from build123d import *

# Parameters (mm, degrees)
BOX019_W               = 120
BOX019_H               = 30
BOX019_DEPTH           = 120
CYLINDER075_R          = 2.5
CYLINDER075_DEPTH      = 10
CYLINDER076_R          = 2.5
CYLINDER076_DEPTH      = 10
CYLINDER077_R          = 2.5
CYLINDER077_DEPTH      = 10
CYLINDER078_R          = 2.5
CYLINDER078_DEPTH      = 10
CYLINDER074_R          = 2.5
CYLINDER074_DEPTH      = 10
CYLINDER079_R          = 2.5
CYLINDER079_DEPTH      = 10
BOX016_W               = 240
BOX016_H               = 5
BOX016_DEPTH           = 24
BOX017_W               = 140
BOX017_H               = 5
BOX017_DEPTH           = 38
BOX018_W               = 140
BOX018_H               = 5
BOX018_DEPTH           = 77
CUT010_PLACEMENT_ANGLE = 270


with BuildPart() as gatewaycut002:
    # Box019 → Box019 (new body)
    with BuildSketch(Plane(origin=(-75, -3.2, -111), x_dir=(1, 0, 0), z_dir=(0, 0, 1))):
        with Locations((60, 15)):
            Rectangle(BOX019_W, BOX019_H)
    extrude(amount=BOX019_DEPTH)


with BuildPart() as cylinder075:
    # Cylinder075 → Cylinder075 (new body)
    with BuildSketch(Plane(origin=(115, 0, -31), x_dir=(1, 0, 0), z_dir=(0, -1, 0))):
        Circle(CYLINDER075_R)
    extrude(amount=CYLINDER075_DEPTH)


with BuildPart() as cylinder076:
    # Cylinder076 → Cylinder076 (new body)
    with BuildSketch(Plane(origin=(-80, 0, -31), x_dir=(1, 0, 0), z_dir=(0, -1, 0))):
        Circle(CYLINDER076_R)
    extrude(amount=CYLINDER076_DEPTH)


with BuildPart() as cylinder077:
    # Cylinder077 → Cylinder077 (new body)
    with BuildSketch(Plane(origin=(50, 0, -31), x_dir=(1, 0, 0), z_dir=(0, -1, 0))):
        Circle(CYLINDER077_R)
    extrude(amount=CYLINDER077_DEPTH)


with BuildPart() as cylinder078:
    # Cylinder078 → Cylinder078 (new body)
    with BuildSketch(Plane(origin=(-45.75, 0, -56.3), x_dir=(1, 0, 0), z_dir=(0, -1, 0))):
        Circle(CYLINDER078_R)
    extrude(amount=CYLINDER078_DEPTH)


with BuildPart() as cylinder074:
    # Cylinder074 → Cylinder074 (new body)
    with BuildSketch(Plane(origin=(-115, 0, -31), x_dir=(1, 0, 0), z_dir=(0, -1, 0))):
        Circle(CYLINDER074_R)
    extrude(amount=CYLINDER074_DEPTH)


with BuildPart() as m3heatsetinserts004:
    # Cylinder079 → Cylinder079 (new body)
    with BuildSketch(Plane(origin=(-45.75, 0, -1.3), x_dir=(1, 0, 0), z_dir=(0, -1, 0))):
        Circle(CYLINDER079_R)
    extrude(amount=CYLINDER079_DEPTH)

    # Fusion028: union Cylinder075, Cylinder076, Cylinder077, Cylinder078, Cylinder074
    add(cylinder075.part)
    add(cylinder076.part)
    add(cylinder077.part)
    add(cylinder078.part)
    add(cylinder074.part)


with BuildPart() as m3heatsetinserts004_1:
    # Fusion028 placement: moved
    add(m3heatsetinserts004.part.moved(Location((0, 5.1, 0))))


with BuildPart() as cube013:
    # Box016 → Box016 (new body)
    with BuildSketch(Plane(origin=(-120, 0, -43), x_dir=(1, 0, 0), z_dir=(0, 0, 1))):
        with Locations((120, 2.5)):
            Rectangle(BOX016_W, BOX016_H)
    extrude(amount=BOX016_DEPTH)


with BuildPart() as cube014:
    # Box017 → Box017 (new body)
    with BuildSketch(Plane(origin=(-85, 0, -19), x_dir=(1, 0, 0), z_dir=(0, 0, 1))):
        with Locations((70, 2.5)):
            Rectangle(BOX017_W, BOX017_H)
    extrude(amount=BOX017_DEPTH)


with BuildPart() as obj1:
    # Box018 → Box018 (new body)
    with BuildSketch(Plane(origin=(-85, 0, -120), x_dir=(1, 0, 0), z_dir=(0, 0, 1))):
        with Locations((70, 2.5)):
            Rectangle(BOX018_W, BOX018_H)
    extrude(amount=BOX018_DEPTH)

    # Fusion027: union Cube013, Cube014
    add(cube013.part)
    add(cube014.part)

    # Cut009: cut M3HeatSetInserts004
    add(m3heatsetinserts004_1.part, mode=Mode.SUBTRACT)

    # Cut010: cut GatewayCut002
    add(gatewaycut002.part, mode=Mode.SUBTRACT)


with BuildPart() as obj1_1:
    # Cut010 placement: moved
    add(obj1.part.rotate(Axis((0, 0, 0), (1, 0, 0)), CUT010_PLACEMENT_ANGLE))


solid = obj1_1.part
Source: CAD feature listing. Evaluate the final solid. Frame: model axes, mm. A direction names the side the tool comes from. Round coordinates to 2 decimals unless told otherwise and drop trailing zeros. Loops run counter-clockwise (first coordinate to the right, second up) from the corner with the lowest first, then second, coordinate; pieces in that order, holes last.
Q1. Access query for faces 4 (the face through (55, -82, -2)), 5 (the face through (45, -52, -2)), 6 (the face through (-85, -82, -2)). Directions: +Z, -Z, +X, -X, +Y, -Y. A direction counts if a zero-diameter tool reaches every point of the face in a straight line with its end or side. Return the directions, or none.
Q2. Mould query, pull axis Y, two halves, no side actions, for faces 1 (the face through (55, 0, -2)), 2 (the face through (-103, -43, -3)), 3 (the face through (51.34, -28.89, -2.53)). Classes: pulls with the +Y half, pulls with the -Y half, needs draft (parallel to the pull), parting line crosses it, or undercut.
Q3. Section C-C, the plane y = -31. Return loops of the section in (x, z), plus the area to 3 significant figures.
Q4. Section A-A, the plane x = 50. Return loops of the section in (y, z), plus the area to 3 significant figures.
Q5. Section D-D, the plane z = -0.8. Return loops of the section in (x, y).
Q6. Ray query, line 1 (X direction, y = -31, z = -3.15); line 2 (X direction, y = -100, z = -0.6); line 3 (Y direction, x = -42.5, z = -2). Return the intervals inside material, ascending.
Q7. First-contact query: P1, Ø6.5, axis at x = 115, y = -31, coming from the +Z side; P2, Ø4.5, axis at x = -115, y = -31, coming from the -Z side; P3, Ø3, axis at y = -63, z = -0.5, coming from the +X side; P4, Ø1.5, axis at x = 103.5, z = -1.5, coming from the -Y side. Flat tips, straight axial feed; report the tip coordinate or a pass-through.
Q8. Section B-B, the plane y = 1. Return loops of the section in (x, z).
Solutions:
1. face 4: +Z, -Z, +X, -Y
1. face 5: +Z, -Z
1. face 6: +Z, -Z, -X, -Y
2. face 1: needs draft
2. face 2: pulls with the -Y half
2. face 3: undercut
3. outline: (-120, -5) - (-117.5, -5) - (-117.5, 0) - (-120, 0) - close; (-112.5, -5) - (-82.5, -5) - (-82.5, 0) - (-112.5, 0) - close; (-77.5, -5) - (-75, -5) - (-75, 0) - (-77.5, 0) - close; (45, -5) - (47.5, -5) - (47.5, 0) - (45, 0) - close; (52.5, -5) - (112.5, -5) - (112.5, 0) - (52.5, 0) - close; (117.5, -5) - (120, -5) - (120, 0) - (117.5, 0) - close
3. area: 500 mm2
4. outline: (-120, -5) - (-33.5, -5) - (-33.5, 0) - (-120, 0) - close; (-28.5, -5) - (19, -5) - (19, 0) - (-28.5, 0) - close
4. area: 670 mm2
5. outline: (-120, -43) - (-85, -43) - (-85, -120) - (55, -120) - (55, -43) - (120, -43) - (120, -19) - (55, -19) - (55, 19) - (-85, 19) - (-85, -19) - (-120, -19) - close; hole circle Ø5 at (-115, -31); hole circle Ø5 at (-80, -31); hole (-75, -111) - (45, -111) - (45, 9) - (-75, 9) - close; hole circle Ø5 at (50, -31); hole circle Ø5 at (115, -31)
6. line 1: x = -120 to -117.5, -112.5 to -82.5, -77.5 to -75, 45 to 47.5, 52.5 to 112.5, 117.5 to 120
6. line 2: x = -85 to -75, 45 to 55
6. line 3: y = -120 to -111, 9 to 19
7. P1: stops at z = 0
7. P2: passes through
7. P3: stops at x = 55
7. P4: stops at y = -43
8. outline: (-85, -5) - (-75, -5) - (-75, 0) - (-85, 0) - close; (45, -5) - (55, -5) - (55, 0) - (45, 0) - close
